Verification items for the finished model (mm, model axes). A direction names the side the tool comes from. Round coordinates to 2 decimals unless told otherwise and drop trailing zeros. Order: outer loops, then holes, each group sorted by start corner. A loop starts at its lowest first (then second) coordinate and runs counter-clockwise, first axis right, second up. Notation, with made-up numbers: (0, -21.5) -> (9, -21.5) arc R6 ccw to (9, -16.5) -> close; hole circle Ø3 at (87, 23.25). An arc over 180 degrees is marked (long way). Put each result on its own line as item: value.
```python
from build123d import *

# Parameters (mm, degrees)
SKETCH1_W           = 20
SKETCH1_H           = 30
BOSS_EXTRUDE1_DEPTH = 10
BOSS_EXTRUDE2_DEPTH = 10
SKETCH4_R           = 8.55
BOSS_EXTRUDE3_DEPTH = 10
CUT_EXTRUDE1_DEPTH  = 10
BOSS_EXTRUDE4_DEPTH = 10
SKETCH7_R           = 1.25
CUT_EXTRUDE2_DEPTH  = 10
FILLET1_R           = 5


with BuildPart() as part:
    # Sketch1 → Boss-Extrude1 (new body)
    with BuildSketch(Plane(origin=(0, 0, 0), x_dir=(1, 0, 0), z_dir=(0, 1, 0))):
        with Locations((10, -15)):
            Rectangle(SKETCH1_W, SKETCH1_H)
    extrude(amount=BOSS_EXTRUDE1_DEPTH)

    # Sketch2 → Boss-Extrude2 (add)
    with BuildSketch(Plane(origin=(0, 10, 0), x_dir=(1, 0, 0), z_dir=(0, 1, 0))):
        Polygon((0, 0), (0, -10), (10, -10), (10, -30), (20, -30), (20, 0), align=None)
    boss_extrude2 = extrude(amount=BOSS_EXTRUDE2_DEPTH)

    # Sketch4 → Boss-Extrude3 (add)
    with BuildSketch(Plane(origin=(0, 10, 0), x_dir=(1, 0, 0), z_dir=(0, 1, 0))):
        with BuildLine():
            Line((0, 0), (-17.51372228, 3.319944561))
            ThreePointArc((-17.51372228, 3.319944561), (-33.173842638, -6.829452704), (-23.846362702, -22.992613054))
            Line((-23.846362702, -22.992613054), (0, -30))
            Line((0, -30), (0, 0))
        make_face()
        with Locations(Location((-20, -10, 0), (0, 0, 270))):
            Circle(SKETCH4_R, mode=Mode.SUBTRACT)
    extrude(amount=-BOSS_EXTRUDE3_DEPTH)

    # Mirror1: Boss-Extrude2 across plane
    add(boss_extrude2.mirror(Plane(origin=(0, 5, 0), x_dir=(0, 0, 1), z_dir=(0, -1, 0))))

    # Sketch5 → Cut-Extrude1 (cut)
    with BuildSketch(Plane(origin=(0, 20, 0), x_dir=(1, 0, 0), z_dir=(0, 1, 0))):
        Polygon((20, 0), (0, 0), (0, -10), (10, -10), (10, -30), (20, -30), align=None)
    extrude(amount=-CUT_EXTRUDE1_DEPTH, mode=Mode.SUBTRACT)

    # Sketch6 → Boss-Extrude4 (add)
    with BuildSketch(Plane.XZ.offset(10)):
        Polygon((0, 0), (20, 0), (20, 30), (10, 30), (10, 10), (0, 10), align=None)
    extrude(amount=BOSS_EXTRUDE4_DEPTH)

    # Sketch7 → Cut-Extrude2 (cut)
    with BuildSketch(Plane.ZY.offset(-10)):
        with Locations((20, -10)):
            Circle(SKETCH7_R)
    extrude(amount=-CUT_EXTRUDE2_DEPTH, mode=Mode.SUBTRACT)

    # Fillet1
    fillet1_edges = [part.edges().sort_by_distance(p)[0] for p in [
        (20, -5, 0),
        (20, -5, 30),
        (20, 10, 15),
    ]]
    fillet(fillet1_edges, radius=FILLET1_R)


solid = part.part
```
Item 1: Sectioned sample at C-C, the plane y = -10. Record the boundary of the cut face in (x, z), then the cut area to 3 significant figures.
Geometry check:
outline: (0, 0) -> (15, 0) arc R5 ccw to (20, 5) -> (20, 18.75) -> (10, 18.75) -> (10, 10) -> (0, 10) -> close; (10, 21.25) -> (20, 21.25) -> (20, 25) arc R5 ccw to (15, 30) -> (10, 30) -> close
area: 364 mm2
Item 2: Release check for a two-part mould opening along Z. For faces 1 (the face through (11, -1, 30)), 2 (the face through (14.93, -9.62, 21.19)), 3 (the face through (-7, 0, 13)) record: pulls with the +Z half, pulls with the -Z half, needs draft (parallel to the pull), parting line crosses it, or undercut.
Geometry check:
face 1: pulls with the +Z half
face 2: undercut
face 3: needs draft
Item 3: Material ranges on line 1 along Y through (x, z) = (12.75, 20); line 2 along X through (y, z) = (2.5, 10); line 3 along X through (y, z) = (6, 10), recorded low to high.
Geometry check:
line 1: -20 to -11.25, -8.75 to 10
line 2: -33.55 to -28.55, -11.45 to 20
line 3: -33.55 to -28.55, -11.45 to 19.9
Item 4: Sectioned sample at B-B, the plane z = 20. Record the boundary of the cut face in (x, y), then the cut area to 3 significant figures.
Geometry check:
outline: (-29.14, 0) -> (10, 0) -> (10, -8.75) -> (20, -8.75) -> (20, 5) arc R5 ccw to (15, 10) -> (-29.14, 10) -> close; (10, -20) -> (20, -20) -> (20, -11.25) -> (10, -11.25) -> close
area: 661 mm2
Item 5: Tool access check on faces 4 (the face through (0, -10, 5)), 5 (the face through (10, -10, 22)), 6 (the face through (7, -5, 0)). Record the directions out of +Z, -Z, +X, -X, +Y, -Y that give a thin tool (end or side, any length) a straight path to the whole face; none if there is none.
Geometry check:
face 4: +Z, -Z, -X, -Y
face 5: +Z, -X, -Y
face 6: -Z, +X, +Y, -Y
Item 6: Sectioned sample at D-D, the plane x = 1.5. Record the boundary of the cut face in (y, z), then the cut area to 3 significant figures.
Geometry check:
outline: (-20, 0) -> (10, 0) -> (10, 30) -> (0, 30) -> (0, 10) -> (-20, 10) -> close
area: 500 mm2
Item 7: Sectioned sample at A-A, the plane y = 2.5. Record the boundary of the cut face in (x, z).
Geometry check:
outline: (-23.85, 22.99) arc R13.55 ccw to (-17.51, -3.32) -> (0, 0) -> (15, 0) arc R5 ccw to (20, 5) -> (20, 25) arc R5 ccw to (15, 30) -> (0, 30) -> close; hole circle Ø17.1 at (-20, 10)
Item 8: Depth check by flat-ended pin: pin 1 Ø10 at (y, z) = (-9, 23.5) entering from -X; pin 2 Ø3 at (x, y) = (8, -12) entering from -Z; pin 3 Ø2 at (x, y) = (-5, 3) entering from +Z; pin 4 Ø15.5 at (x, z) = (-20, 10) entering from +Y. Enter the tip coordinate at first touch or a pass-through.
Geometry check:
pin 1: x = 10
pin 2: z = 0
pin 3: z = 28.82
pin 4: through
